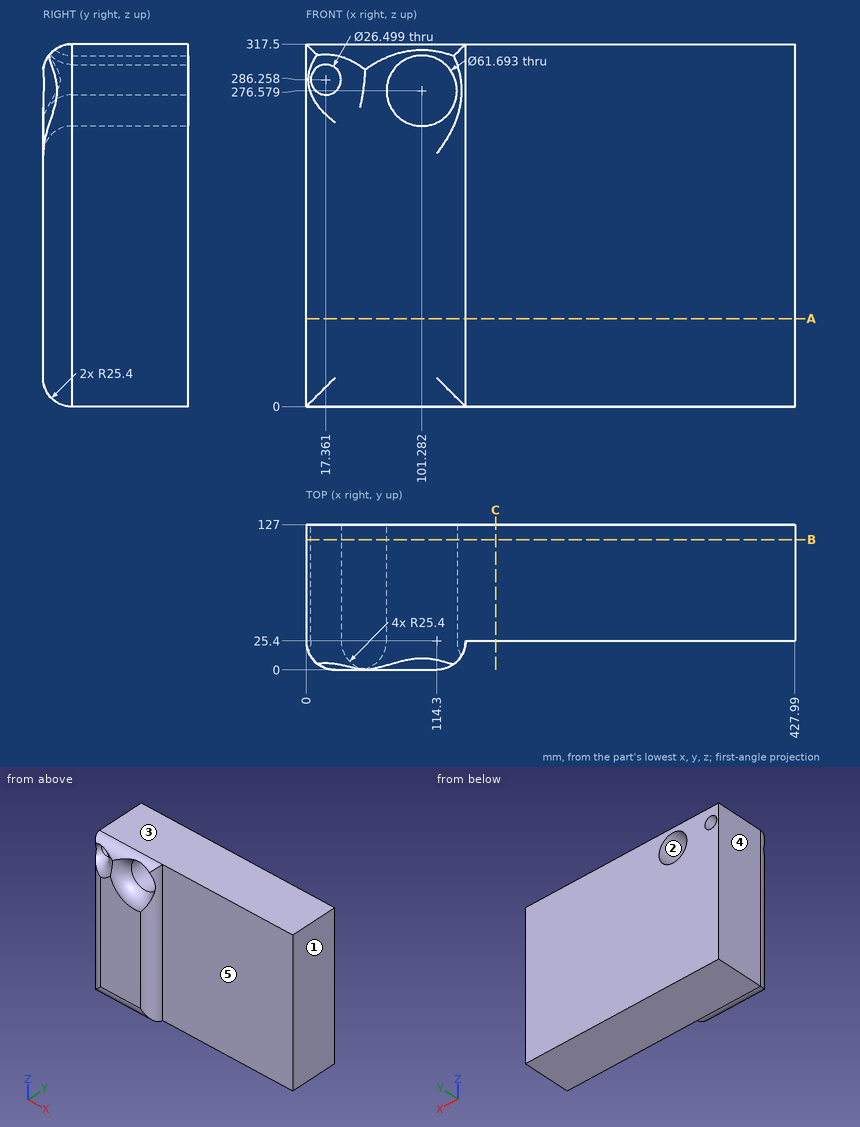
Here's the drawing with two shaded views (mm, measured from the low corner). I have some questions. A direction names the side the tool comes from. Coordinates: 2 decimals unless noted, no trailing zeros. Write each loop counter-clockwise with the first axis right and the second up, starting at its lowest first coordinate (ties: lowest second). Pieces come first, ordered by that corner, then holes. Notation, with made-up numbers: (53, -20) -> (60, -20) arc R28 ccw to (60, 17) -> close; hole circle Ø8 at (65.5, 75). An arc over 180 degrees is marked (long way). Use a Markdown table: item, result. Add a question column.
(1) Please list where these lines run through material, in increasing order: line 1 (Y direction, x = 321, z = 222); line 2 (Z direction, x = 104, y = 55) (1 decimal); line 3 (Z direction, x = 77.5, y = 106) (1 decimal).
(2) For the marked faces 4 and 5, which set-ups out of +Z, -Z, +X, -X, +Y, -Y let a thin tool reach every point of the face, with its end or its side?
(3) If we section it at B-B, the plane y = 114: Write out the boundary of the cut face in (x, z).
(4) I'm going to push flat-ended pins straight in: P1, Ø4, axis at x = 164, z = 123.5, coming from the -Y side; P2, Ø16, axis at x = 17.36, z = 286.26, coming from the +Y side. Where does each tip first touch, or does it pass through?
(5) If we section it at A-A, the plane z = 77: Write out the boundary of the cut face in (x, y).
(6) We'd pull the mould along X, two halves only. Please class the marked faces 1, 2 and 3: +X half, -X half, draft (parallel to the pull), parting line (faces both ways), or undercut.
(7) If we section it at C-C, the plane x = 166: Write out the boundary of the cut face in (y, z).
Outcome:
| question | item | result |
|---|---|---|
| 1 | line 1 | y = 25.4 to 127 |
| 1 | line 2 | z = 0 to 245.9, 307.3 to 317.5 |
| 1 | line 3 | z = 0 to 256.9, 296.2 to 317.5 |
| 2 | face 4 | +Z, -Z, -X, +Y, -Y |
| 2 | face 5 | +Z, -Z, +X, -Y |
| 3 | outline | (0, 0) -> (427.99, 0) -> (427.99, 317.5) -> (0, 317.5) -> close; hole circle Ø26.5 at (17.36, 286.26); hole circle Ø61.69 at (101.28, 276.58) |
| 4 | P1 | stops at y = 25.4 |
| 4 | P2 | passes through |
| 5 | outline | (0, 25.4) arc R25.4 ccw to (25.4, 0) -> (114.3, 0) arc R25.4 ccw to (139.7, 25.4) -> (427.99, 25.4) -> (427.99, 127) -> (0, 127) -> close |
| 6 | face 1 | +X half |
| 6 | face 2 | undercut |
| 6 | face 3 | draft |
| 7 | outline | (25.4, 0) -> (127, 0) -> (127, 317.5) -> (25.4, 317.5) -> close |
